from build123d import *

# Parameters (mm, degrees)
F1_DEPTH = 95.25


with BuildPart() as f1:
    # F0 (on Right) → F1 (new body)
    with BuildSketch(Plane.YZ):
        with BuildLine():
            ThreePointArc((22.225, 7.239), (21.555446, 8.855446), (19.939, 9.525))
            ThreePointArc((19.939, 9.525), (18.619177, 9.105511), (17.783739, 8.001))
            ThreePointArc((17.783739, 8.001), (19.552433, 4.985922), (22.225, 7.239))
        make_face()
        with BuildLine():
            ThreePointArc((17.783739, 8.001), (18.619177, 9.105511), (19.939, 9.525))
            Line((19.939, 9.525), (-22.225, 9.525))
            Line((-22.225, 9.525), (-22.225, -9.525))
            Line((-22.225, -9.525), (-20.701, -9.525))
            Line((-20.701, -9.525), (-20.701, 8.001))
            Line((-20.701, 8.001), (17.783739, 8.001))
        make_face()
    extrude(amount=F1_DEPTH)


solid = f1.part
For this review, take the finished solid that the model builds, in its own axes (mm). A direction names the side the tool comes from. Coordinates: 2 decimals unless noted, no trailing zeros. Order: outer loops, then holes, each group sorted by start corner. A loop starts at its lowest first (then second) coordinate and runs counter-clockwise, first axis right, second up. Notation, with made-up numbers: (69, -37.5) -> (76, -37.5) arc R28 cw to (76, 0.5) -> close; hole circle Ø1 at (-12.5, 8). An arc over 180 degrees is marked (long way). Return JSON: item names as keys, results as strings.
1. For line 1 (Y direction, x = 27, z = 7) (3 decimals); line 2 (Z direction, x = 23.5, y = 13) (3 decimals); line 3 (Y direction, x = 60, z = -5) (3 decimals), list the stretches that pass through material, from the lowest coordinate up. Write a range as from..to.
Answer block:
{"line 1": "-22.225..-20.701, 17.666..22.212", "line 2": "8.001..9.525", "line 3": "-22.225..-20.701"}
2. We need section C-C on y = 5.5. Write out the cut boundary in (x, z) (3 decimals), and give its area (3 significant figures).
Answer block:
{"outline": "(0, 8.001) -> (95.25, 8.001) -> (95.25, 9.525) -> (0, 9.525) -> close", "area": "145 mm²"}
3. We need section A-A on x = 77. Write out the cut boundary in (y, z) (3 decimals).
Answer block:
{"outline": "(-22.225, -9.525) -> (-20.701, -9.525) -> (-20.701, 8.001) -> (17.784, 8.001) arc R2.286 ccw (long way) to (19.939, 9.525) -> (-22.225, 9.525) -> close"}
4. We need section B-B on z = -3.75. Write out the cut boundary in (x, y) (3 decimals), and give its area (3 significant figures).
Answer block:
{"outline": "(0, -22.225) -> (95.25, -22.225) -> (95.25, -20.701) -> (0, -20.701) -> close", "area": "145 mm²"}
5. Machinability: for faces 4 (the flat face through (47, -20.701, -1)), 5 (the flat face through (95.25, -3, 9)), which of the approach directions +Z, -Z, +X, -X, +Y, -Y give a long, thin tool a straight path to every point of the face, cutting with its end or side? Answer none if there is none.
Answer block:
{"face 4": "-Z, +X, -X", "face 5": "+Z, -Z, +X, +Y, -Y"}
6. The part is to be moulded in two halves that separate along Y. For faces 1 (the flat face through (47, -2, 8.001)), 2 (the flat face through (47, -22.225, 0)), 3 (the flat face through (0, -3, 9)), say which applies: +Y half, -Y half, draft (parallel to the pull), parting line (faces both ways), or undercut.
Answer block:
{"face 1": "undercut", "face 2": "-Y half", "face 3": "draft"}
7. For pin 1 Ø10 at (y, z) = (-6, 3.5) entering from -X; pin 2 Ø10 at (x, y) = (40, 3) entering from -Z; pin 3 Ø4 at (x, z) = (78.5, 0) entering from +Y, all flat-tipped, find the tip position at first contact; note any pin that passes through.
Answer block:
{"pin 1": "x = 0", "pin 2": "z = 8", "pin 3": "y = -20.7"}
